For this review, use the dimensioned drawing (mm, ordinates from the lowest corner) and the shaded views. Coordinates: 2 decimals unless noted, no trailing zeros. Write each loop counter-clockwise with the first axis right and the second up, starting at its lowest first coordinate (ties: lowest second). Pieces come first, ordered by that corner, then holes. Notation, with made-up numbers: M 2,-36 L 32,-36 A35 cw 32,-2 Z; hole C 49,19.5 d4. An arc over 180 degrees is marked long. One line per question, with ' | ' between items.
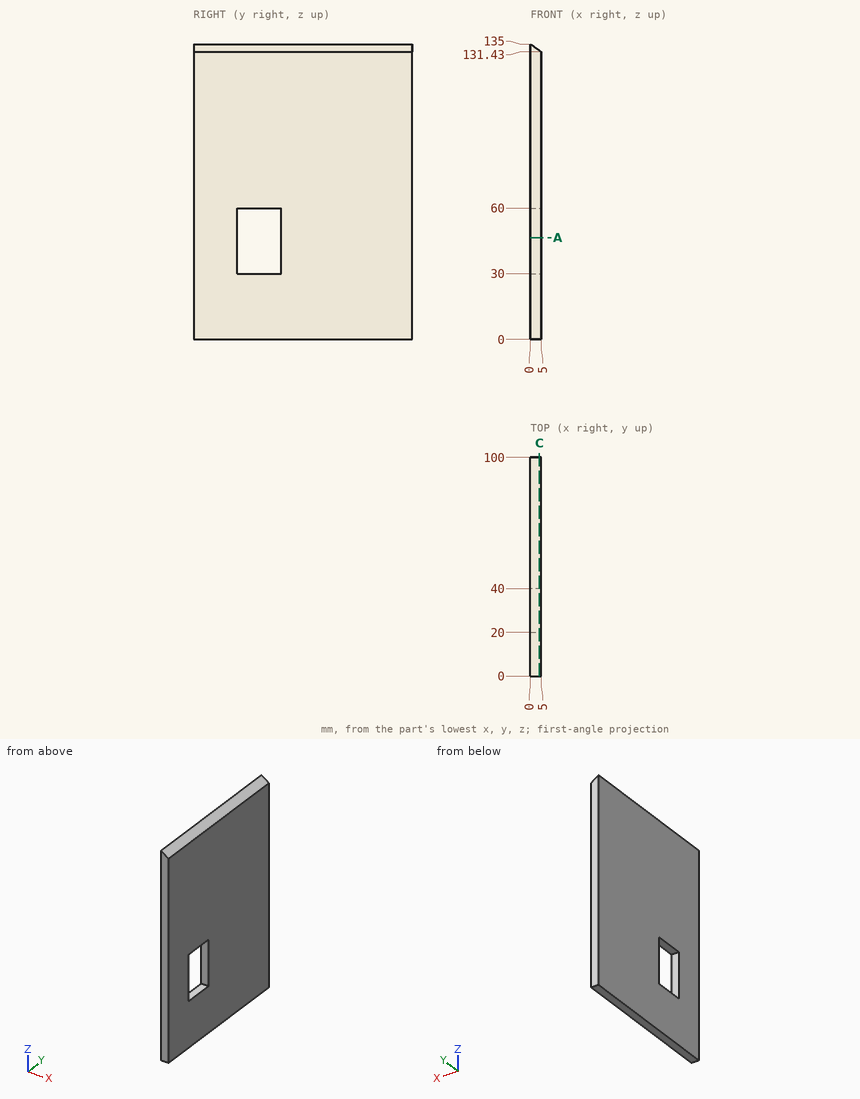
1) To check wall thickness, follow line 1 along Z through (x, y) = (3.05, 34.5); line 2 along Z through (x, y) = (1.65, 83); line 3 along Z through (x, y) = (2.1, 6.5). State the ranges of each line that lie inside material, in increasing order. Write a range as [from, to].
Responses:
line 1: [0, 30], [60, 132.82] | line 2: [0, 133.82] | line 3: [0, 133.5]
2) We need section C-C on x = 4.1. State the section outline as (y, z) points.
Responses:
outline: M 0,0 L 100,0 L 100,132.07 L 0,132.07 Z; hole M 20,30 L 40,30 L 40,60 L 20,60 Z
3) We need section A-A on z = 46.5. State the section outline as (x, y) points, then the cut area to 3 significant figures.
Responses:
outline: M 0,0 L 5,0 L 5,20 L 0,20 Z; M 0,40 L 5,40 L 5,100 L 0,100 Z | area: 400 mm^2
